from build123d import *

# Parameters (mm, degrees)
CROQUIS1_R              = 4
SALIENTE_EXTRUIR1_DEPTH = 10
CROQUIS2_R              = 5
CROQUIS2_R_2            = 2.5
SALIENTE_EXTRUIR2_DEPTH = 18


with BuildPart() as part:
    # Croquis1 → Saliente-Extruir1 (new body)
    with BuildSketch(Plane.XY):
        with BuildLine():
            Line((60.267364884, 6), (-9.732635116, 6))
            ThreePointArc((-9.732635116, 6), (-15.732635116, 0), (-9.732635116, -6))
            Line((-9.732635116, -6), (60.267364884, -6))
            ThreePointArc((60.267364884, -6), (66.267364884, 0), (60.267364884, 6))
        make_face()
        with Locations((-9.732635116, 0)):
            Circle(CROQUIS1_R, mode=Mode.SUBTRACT)
    extrude(amount=SALIENTE_EXTRUIR1_DEPTH)

    # Croquis2 → Saliente-Extruir2 (add)
    with BuildSketch(Plane.XY.offset(10)):
        with Locations((60.267364884, 0)):
            Circle(CROQUIS2_R)
        with Locations((60.267364884, 0)):
            Circle(CROQUIS2_R_2, mode=Mode.SUBTRACT)
    extrude(amount=SALIENTE_EXTRUIR2_DEPTH)


solid = part.part
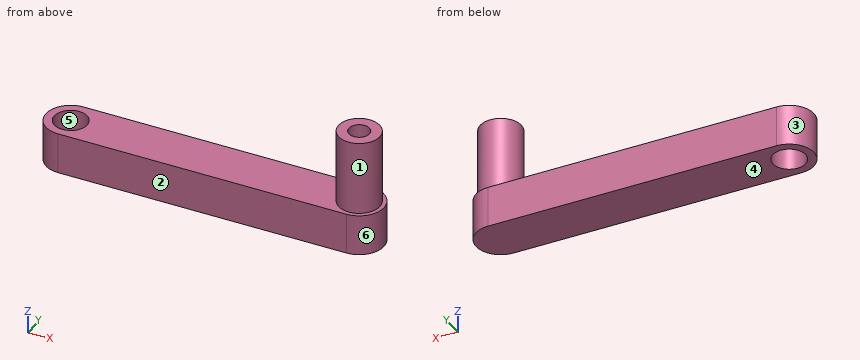
Design review of the part built by this model. Coordinates are the model's own, in mm. Face numbers are marked on the shaded views. A direction names the side the tool comes from. Coordinates: 2 decimals unless noted, no trailing zeros. Write each loop counter-clockwise with the first axis right and the second up, starting at its lowest first coordinate (ties: lowest second). Pieces come first, ordered by that corner, then holes. Notation, with made-up numbers: (34.25, 80.5) - (78.25, 80.5) arc R29 cw to (78.25, 112.5) - close; hole circle Ø4 at (-28, -9.75). An arc over 180 degrees is marked (long way). One line per item, written item: value.
1) To check wall thickness, follow probe 1 along Z at (x, y) = (5.5, -2.25); probe 2 along X at (y, z) = (-0.5, 9.5); probe 3 along X at (y, z) = (-1.75, 25). State the ranges of each line that lie inside material, in increasing order.
Answer sheet:
probe 1: z = 0 to 10
probe 2: x = -15.71 to -13.7, -5.76 to 66.25
probe 3: x = 55.58 to 58.48, 62.05 to 64.95
2) Add section D-D (x = 8.5). State the section outline as (y, z) points, plus the area to 3 significant figures.
Answer sheet:
outline: (-6, 0) - (6, 0) - (6, 10) - (-6, 10) - close
area: 120 mm2
3) Add section B-B (z = 8.25). State the section outline as (x, y) points, plus the area to 3 significant figures.
Answer sheet:
outline: (-9.73, -6) - (60.27, -6) arc R6 ccw to (60.27, 6) - (-9.73, 6) arc R6 ccw to start; hole circle Ø8 at (-9.73, 0)
area: 903 mm2
4) For the marked faces 1 and 2, list the 3-axis set-ups (+Z, -Z, +X, -X, +Y, -Y) from which the entire face can be reached by the end or side of a thin tool; tool diameter is ignored.
Answer sheet:
face 1: +Z
face 2: +Z, -Z, +X, -X, -Y
5) Add section C-C (y = -3.25). State the section outline as (x, z) points.
Answer sheet:
outline: (-14.78, 0) - (-12.06, 0) - (-12.06, 10) - (-14.78, 10) - close; (-7.4, 0) - (65.31, 0) - (65.31, 10) - (64.07, 10) - (64.07, 28) - (56.47, 28) - (56.47, 10) - (-7.4, 10) - close
6) Add section A-A (y = 0). State the section outline as (x, z) points, plus the area to 3 significant figures.
Answer sheet:
outline: (-15.73, 0) - (-13.73, 0) - (-13.73, 10) - (-15.73, 10) - close; (-5.73, 0) - (66.27, 0) - (66.27, 10) - (65.27, 10) - (65.27, 28) - (62.77, 28) - (62.77, 10) - (57.77, 10) - (57.77, 28) - (55.27, 28) - (55.27, 10) - (-5.73, 10) - close
area: 830 mm2
7) Mouldability with a two-part tool opening along X and no side actions: class the marked faces 3, 4, 5 and 6 as +X half, -X half, draft (parallel to the pull), parting line (faces both ways), or undercut.
Answer sheet:
face 3: -X half
face 4: draft
face 5: undercut
face 6: +X half
8) Insertion check: pin 1 (4 mm diameter, centred on y = -3.5, z = 8, fed in from -X); pin 2 (1.5 mm diameter, centred on y = 2.5, z = 18, fed in from -X); pin 3 (3.5 mm diameter, centred on x = 23, y = 0.5, fed in from +Z). Each pin has a flat end and moves straight along its axis. Give the tip position at first contact, or say it passes through.
Answer sheet:
pin 1: stops at x = -15.54
pin 2: stops at x = 55.58
pin 3: stops at z = 10
